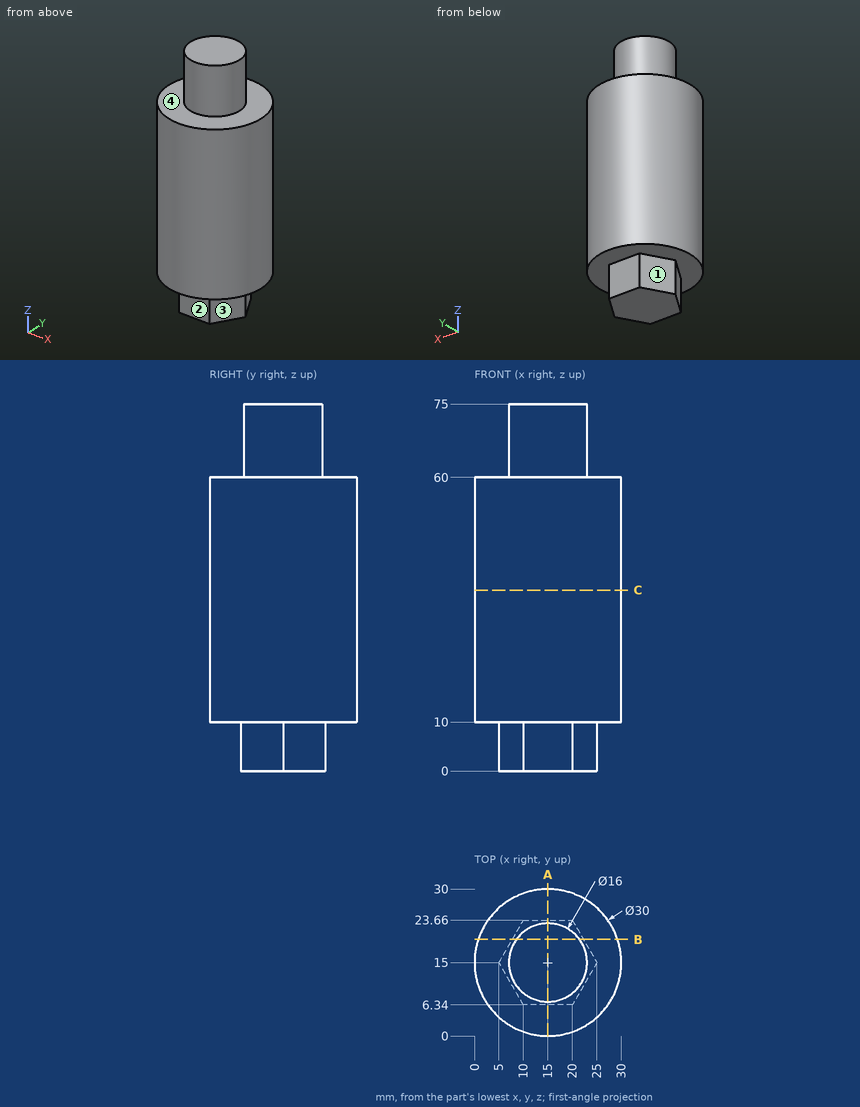
Print and shaded views of the part. All mm, measured from the part's lowest x, y and z. A direction names the side the tool comes from. Coordinates: 2 decimals unless noted, no trailing zeros. Write each loop counter-clockwise with the first axis right and the second up, starting at its lowest first coordinate (ties: lowest second). Pieces come first, ordered by that corner, then holes.
(1) Drill centre lines: probe 1 along Z at (x, y) = (3, 7.25); probe 2 along X at (y, z) = (24.25, 20.5); probe 3 along X at (y, z) = (1.5, 52.5). Where is each one in solid material? Low to high.
(2) Flat gauge pins, fed straight in: pin 1 (10 mm diameter, centred on x = 5, z = 19.5, fed in from -Y); pin 2 (1.5 mm diameter, centred on x = 6, z = 28, fed in from -Y); pin 3 (10 mm diameter, centred on y = 19, z = 32, fed in from -X); pin 4 (5 mm diameter, centred on x = 13.5, z = 6, fed in from +Y). Where does each tip first touch, or does it go through?
(3) Cut at C-C, the plane z = 37. List the corners of the cut face in (x, y), and give its area (3 significant figures).
(4) Cut at A-A, the plane x = 15. List the corners of the cut face in (y, z), and give its area (3 significant figures).
(5) 3-axis set-ups, long thin cutter, end or side, ignore diameter. For the marked faces 1, 2, 3 and 4: which of +Z, -Z, +X, -X, +Y, -Y reach the whole face in a straight line?
(6) Cut at B-B, the plane y = 19.75. List the corners of the cut face in (x, z), and give its area (3 significant figures).
Geometry says:
1. probe 1: z = 10 to 60
1. probe 2: x = 3.19 to 26.81
1. probe 3: x = 8.46 to 21.54
2. pin 1: stops at y = 0.86
2. pin 2: stops at y = 2.47
2. pin 3: stops at x = 0
2. pin 4: stops at y = 23.66
3. outline: circle Ø30 at (15, 15)
3. area: 707 mm2
4. outline: (0, 10) - (6.34, 10) - (6.34, 0) - (23.66, 0) - (23.66, 10) - (30, 10) - (30, 60) - (23, 60) - (23, 75) - (7, 75) - (7, 60) - (0, 60) - close
4. area: 1,910 mm2
5. face 1: -Z, -X, +Y
5. face 2: -Z, +X, -X, -Y
5. face 3: -Z, +X, -Y
5. face 4: +Z
6. outline: (0.77, 10) - (7.74, 10) - (7.74, 0) - (22.26, 0) - (22.26, 10) - (29.23, 10) - (29.23, 60) - (21.44, 60) - (21.44, 75) - (8.56, 75) - (8.56, 60) - (0.77, 60) - close
6. area: 1,760 mm2
